For this review, take the finished solid that the model builds, in its own axes (mm). Face numbers are marked on the shaded views. Round coordinates to 2 decimals unless told otherwise and drop trailing zeros. Write each loop counter-clockwise with the first axis right and the second up, starting at its lowest first coordinate (ties: lowest second). Pieces come first, ordered by that corner, then holes. Notation, with made-up numbers: (66, 20.5) -> (108, 20.5) arc R11 cw to (108, 39.5) -> close; hole circle Ø11 at (59, -36). An arc over 180 degrees is marked (long way). Answer as CSV lines item,"result". Start each with the question number.
Item 1: For pin 1 Ø12 at (x, y) = (-132.5, 183.5) entering from -Z; pin 2 Ø12 at (x, y) = (39.5, 25) entering from +Z, all flat-tipped, find the tip position at first contact; note any pin that passes through.
Item 2: Wall thickness on probe 1 along X at (y, z) = (-186.5, 16); probe 2 along Y at (x, z) = (127.5, 27) (3 decimals): over which ranges is each line inside the solid? List them lowest first. Write a range as from..to.
Item 3: Take a section at A-A on z = 27. Give the boundary of the cut face in (x, y) (3 decimals).
Item 4: Take a section at C-C on x = 359. Give the boundary of the cut face in (y, z).
Item 5: Mouldability with a two-part tool opening along Y and no side actions: class the marked faces 1 and 2 as +Y half, -Y half, draft (parallel to the pull), parting line (faces both ways), or undercut.
Item 6: Take a section at D-D on y = 198. Give the boundary of the cut face in (x, z), then the cut area to 3 significant figures.
Item 7: Take a section at B-B on y = -269.5. Give the boundary of the cut face in (x, z), then the cut area to 3 significant figures.
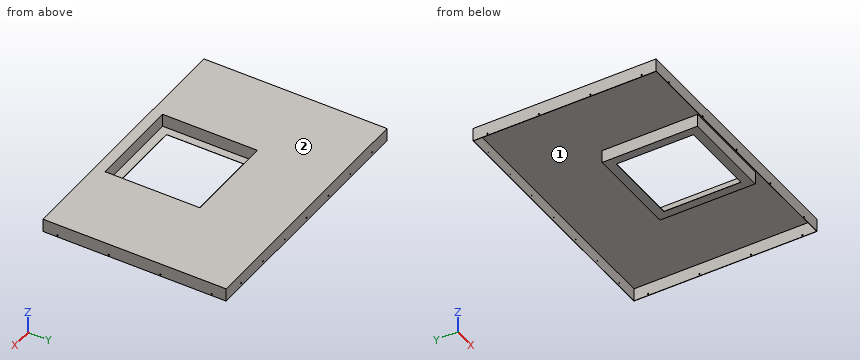
```python
from build123d import *

# Parameters (mm, degrees)
F1_DEPTH  = 52.324
F2_T      = -1.27
F4_D      = 5.2197
F4_DEPTH  = 0.762
F4_TIP    = 1.5681560866
F6_D      = 5.2197
F7_W      = 368.3
F7_H      = 374.65
F8_DEPTH  = 52.325
F9_W      = 369.824
F9_H      = 376.174
F9_W_2    = 368.3
F9_H_2    = 374.65
F10_DEPTH = 51.562
F11_W     = 368.3
F11_H     = 374.65
F11_W_2   = 304.8
F11_H_2   = 304.8
F12_DEPTH = 0.762
F14_D     = 5.2197
F14_DEPTH = 0.762
F14_TIP   = 1.5681560866
F16_D     = 5.2197
F16_DEPTH = 0.762
F16_TIP   = 1.5681560866


with BuildPart() as f1:
    # F0 (on Top) → F1 (new body)
    with BuildSketch(Plane.XY):
        Polygon((-514.35, 361.95), (-514.35, -361.95), (0, -361.95), (0, 0), (0, 361.95), align=None)
        Polygon((0, 0), (0, -361.95), (514.35, -361.95), (514.35, 361.95), (0, 361.95), align=None)
    extrude(amount=F1_DEPTH)

    # F2
    f2_openings = [f1.faces().sort_by_distance(p)[0] for p in [
        (0, 0, 0),
    ]]
    offset(amount=F2_T, openings=f2_openings)

    # F4
    with Locations(Plane.XZ.offset(361.95)):
        with Locations((-431.8, 7.112), (-215.9, 7.112), (0, 7.112), (215.9, 7.112), (431.8, 7.112)):
            Hole(F4_D / 2, depth=F4_DEPTH)
            with Locations((0, 0, -(F4_DEPTH + F4_TIP / 2))):  # 118° drill point
                Cone(0, F4_D / 2, F4_TIP, mode=Mode.SUBTRACT)

    # F6 (through all)
    with Locations(Plane.YZ.offset(514.35)):
        with Locations((-304.8, 7.112), (-101.6, 7.112), (101.6, 7.112), (304.8, 7.112)):
            Hole(F6_D / 2)

    # F7 (on face) → F8 (cut, through all)
    with BuildSketch(Plane.XY.offset(52.324)):
        with Locations((0, -133.35)):
            Rectangle(F7_W, F7_H)
    extrude(amount=-F8_DEPTH, mode=Mode.SUBTRACT)

    # F9 (on face) → F10 (join)
    with BuildSketch(Plane.XY.offset(52.324)):
        with Locations((0, -133.35)):
            Rectangle(F9_W, F9_H)
        with Locations((0, -133.35)):
            Rectangle(F9_W_2, F9_H_2, mode=Mode.SUBTRACT)
    extrude(amount=-F10_DEPTH)

    # F11 (on face) → F12 (join)
    with BuildSketch(Plane(origin=(0, 0, 0.762), x_dir=(1, 0, 0), z_dir=(0, 0, -1))):
        with Locations((0, 133.35)):
            Rectangle(F11_W, F11_H)
        with Locations((0, 133.35)):
            Rectangle(F11_W_2, F11_H_2, mode=Mode.SUBTRACT)
    extrude(amount=-F12_DEPTH)

    # F14
    with Locations(Plane(origin=(0, 361.95, 0), x_dir=(-1, 0, 0), z_dir=(0, 1, 0))):
        with Locations((-419.1, 14.2875), (-279.4, 14.2875), (-139.7, 14.2875), (0, 14.2875), (139.7, 14.2875), (279.4, 14.2875), (419.1, 14.2875)):
            Hole(F14_D / 2, depth=F14_DEPTH)
            with Locations((0, 0, -(F14_DEPTH + F14_TIP / 2))):  # 118° drill point
                Cone(0, F14_D / 2, F14_TIP, mode=Mode.SUBTRACT)

    # F16 (one way)
    with BuildSketch(Plane.XZ.offset(-53.975)):
        with Locations((-127, 38.1), (-63.5, 38.1), (0, 38.1), (63.5, 38.1), (127, 38.1)):
            Circle(F16_D / 2)
    extrude(amount=-F16_DEPTH, mode=Mode.SUBTRACT)
    with Locations(Plane.XZ.offset(-53.975)):
        with Locations((-127, 38.1), (-63.5, 38.1), (0, 38.1), (63.5, 38.1), (127, 38.1)):
            with Locations((0, 0, -(F16_DEPTH + F16_TIP / 2))):  # 118° drill point
                Cone(0, F16_D / 2, F16_TIP, mode=Mode.SUBTRACT)


solid = f1.part
```
Output values:
1,pin 1,"stops at z = 51.05"
1,pin 2,"stops at z = 1.52"
2,probe 1,"x = -514.35..-513.08, -184.91..-184.15, 184.15..184.91, 513.08..514.35"
2,probe 2,"y = -361.95..-360.68, -321.437..-320.675, 53.975..54.737, 360.68..361.95"
3,outline,"(-514.35, -361.95) -> (514.35, -361.95) -> (514.35, 361.95) -> (-514.35, 361.95) -> close; (-184.912, -321.437) -> (184.912, -321.437) -> (184.912, 54.737) -> (-184.912, 54.737) -> close; hole (-513.08, -360.68) -> (513.08, -360.68) -> (513.08, 360.68) -> (-513.08, 360.68) -> close; hole (-184.15, -320.675) -> (184.15, -320.675) -> (184.15, 53.975) -> (-184.15, 53.975) -> close"
4,outline,"(-361.95, 0) -> (-360.68, 0) -> (-360.68, 51.05) -> (360.68, 51.05) -> (360.68, 0) -> (361.95, 0) -> (361.95, 52.32) -> (-361.95, 52.32) -> close"
5,face 1,"undercut"
5,face 2,"draft"
6,outline,"(-514.35, 0) -> (-513.08, 0) -> (-513.08, 51.05) -> (513.08, 51.05) -> (513.08, 0) -> (514.35, 0) -> (514.35, 52.32) -> (-514.35, 52.32) -> close"
6,area,"1,440 mm^2"
7,outline,"(-514.35, 0) -> (-513.08, 0) -> (-513.08, 51.05) -> (-184.91, 51.05) -> (-184.91, 0.76) -> (-152.4, 0.76) -> (-152.4, 1.52) -> (-184.15, 1.52) -> (-184.15, 52.32) -> (-514.35, 52.32) -> close; (152.4, 0.76) -> (184.91, 0.76) -> (184.91, 51.05) -> (513.08, 51.05) -> (513.08, 0) -> (514.35, 0) -> (514.35, 52.32) -> (184.15, 52.32) -> (184.15, 1.52) -> (152.4, 1.52) -> close"
7,area,"1,090 mm^2"
